Read the model definition and answer for the solid it produces. Units are mm, in the model's axes. A direction names the side the tool comes from. Round coordinates to 2 decimals unless told otherwise and drop trailing zeros. Write each loop counter-clockwise with the first axis right and the second up, starting at its lowest first coordinate (ties: lowest second). Pieces come first, ordered by that corner, then holes. Notation, with made-up numbers: (83, 45.5) -> (90, 45.5) arc R16 ccw to (90, 51.5) -> close; hole circle Ø2 at (19, 78). An arc over 180 degrees is marked (long way). Return JSON: item names as keys, results as strings.
from build123d import *

# Parameters (mm, degrees)
SKETCH_1_W          = 9
SKETCH_1_H          = 9
EXTRUDE_1_DEPTH     = 78
SKETCH_2_W          = 7
SKETCH_2_H          = 7
CUT_EXTRUDE_1_DEPTH = 90
SKETCH_3_R          = 1.65
CUT_EXTRUDE_2_DEPTH = 75
SKETCH_4_R          = 2.1
CUT_EXTRUDE_3_DEPTH = 75


with BuildPart() as part:
    # ｽｹｯﾁ1 → ﾎﾞｽ - 押し出し1 (new body)
    with BuildSketch(Plane.XY):
        Rectangle(SKETCH_1_W, SKETCH_1_H)
    extrude(amount=EXTRUDE_1_DEPTH)

    # ｽｹｯﾁ2 → ｶｯﾄ - 押し出し1 (cut)
    with BuildSketch(Plane.XY.offset(78)):
        Rectangle(SKETCH_2_W, SKETCH_2_H)
    extrude(amount=-CUT_EXTRUDE_1_DEPTH, mode=Mode.SUBTRACT)

    # ｽｹｯﾁ3 → ｶｯﾄ - 押し出し2 (cut)
    with BuildSketch(Plane(origin=(0, 4.5, 0), x_dir=(1, 0, 0), z_dir=(0, 1, 0))):
        with Locations((0, -4.5)):
            Circle(SKETCH_3_R)
        with Locations((0, -73.5)):
            Circle(SKETCH_3_R)
    extrude(amount=-CUT_EXTRUDE_2_DEPTH, mode=Mode.SUBTRACT)

    # ｽｹｯﾁ4 → ｶｯﾄ - 押し出し3 (cut)
    with BuildSketch(Plane(origin=(0, 4.5, 0), x_dir=(1, 0, 0), z_dir=(0, 1, 0))):
        with Locations((0, -31)):
            Circle(SKETCH_4_R)
        with Locations((0, -47)):
            Circle(SKETCH_4_R)
    extrude(amount=-CUT_EXTRUDE_3_DEPTH, mode=Mode.SUBTRACT)


solid = part.part
Item 1: Section B-B (z = 47) is taken. Give the vertices of the cut face in (x, y), then the cut area to 3 significant figures.
Worked answers:
{"outline": "(-4.5, -4.5) -> (-2.1, -4.5) -> (-2.1, -3.5) -> (-3.5, -3.5) -> (-3.5, 3.5) -> (-2.1, 3.5) -> (-2.1, 4.5) -> (-4.5, 4.5) -> close; (2.1, -4.5) -> (4.5, -4.5) -> (4.5, 4.5) -> (2.1, 4.5) -> (2.1, 3.5) -> (3.5, 3.5) -> (3.5, -3.5) -> (2.1, -3.5) -> close", "area": "23.6 mm2"}
Item 2: Section A-A (y = 1.25) is taken. Give the vertices of the cut face in (x, z).
Worked answers:
{"outline": "(-4.5, 0) -> (-3.5, 0) -> (-3.5, 78) -> (-4.5, 78) -> close; (3.5, 0) -> (4.5, 0) -> (4.5, 78) -> (3.5, 78) -> close"}
Item 3: A tool of negligible diameter and unlimited length cuts with its end or side. For faces 4 (the flat face through (-4.5, 0, 38)), 5 (the flat face through (0, 3.5, 40)), from which of +Z, -Z, +X, -X, +Y, -Y can it reach the whole face along a straight path? Write none if from no direction.
Worked answers:
{"face 4": "+Z, -Z, -X, +Y, -Y", "face 5": "+Z, -Z"}
Item 4: For a pull along Y with two mould halves and no side action, classify faces 1 (the flat face through (0, -3.5, 40)), 2 (the flat face through (0, -4.5, 38)), 3 (the cylindrical face through (-0.46, -3.99, 33.05)) as released by +Y, released by -Y, zero draft, split by the parting line, or undercut.
Worked answers:
{"face 1": "undercut", "face 2": "released by -Y", "face 3": "zero draft"}
Item 5: A flat-ended cylindrical pin translates along its axis: pin 1 (2.5 mm diameter, centred on x = 0, z = 4.5, fed in from +Y). Find the tip coordinate at first contact, or state that the pin passes through.
Worked answers:
{"pin 1": "passes through"}
Item 6: Section D-D (x = 0) is taken. State how many separate pieces and enclosed holes the cut face has, then the cut area to 3 significant figures.
Worked answers:
{"separate pieces": "10", "enclosed holes": "0", "area": "126 mm2"}
Item 7: Section C-C (z = 8) is taken. Give the vertices of the cut face in (x, y), then the cut area to 3 significant figures.
Worked answers:
{"outline": "(-4.5, -4.5) -> (4.5, -4.5) -> (4.5, 4.5) -> (-4.5, 4.5) -> close; hole (-3.5, -3.5) -> (3.5, -3.5) -> (3.5, 3.5) -> (-3.5, 3.5) -> close", "area": "32.0 mm2"}
Item 8: Straight lines are drawn through the part: L1, parallel to Z at x = 0, y = -3.7; L2, parallel to X at y = 1.25, z = 63. For each, find the intervals that lie inside material, in ascending order. Write a range as [from, to].
Worked answers:
{"L1": "z = [0, 2.85], [6.15, 28.9], [33.1, 44.9], [49.1, 71.85], [75.15, 78]", "L2": "x = [-4.5, -3.5], [3.5, 4.5]"}
